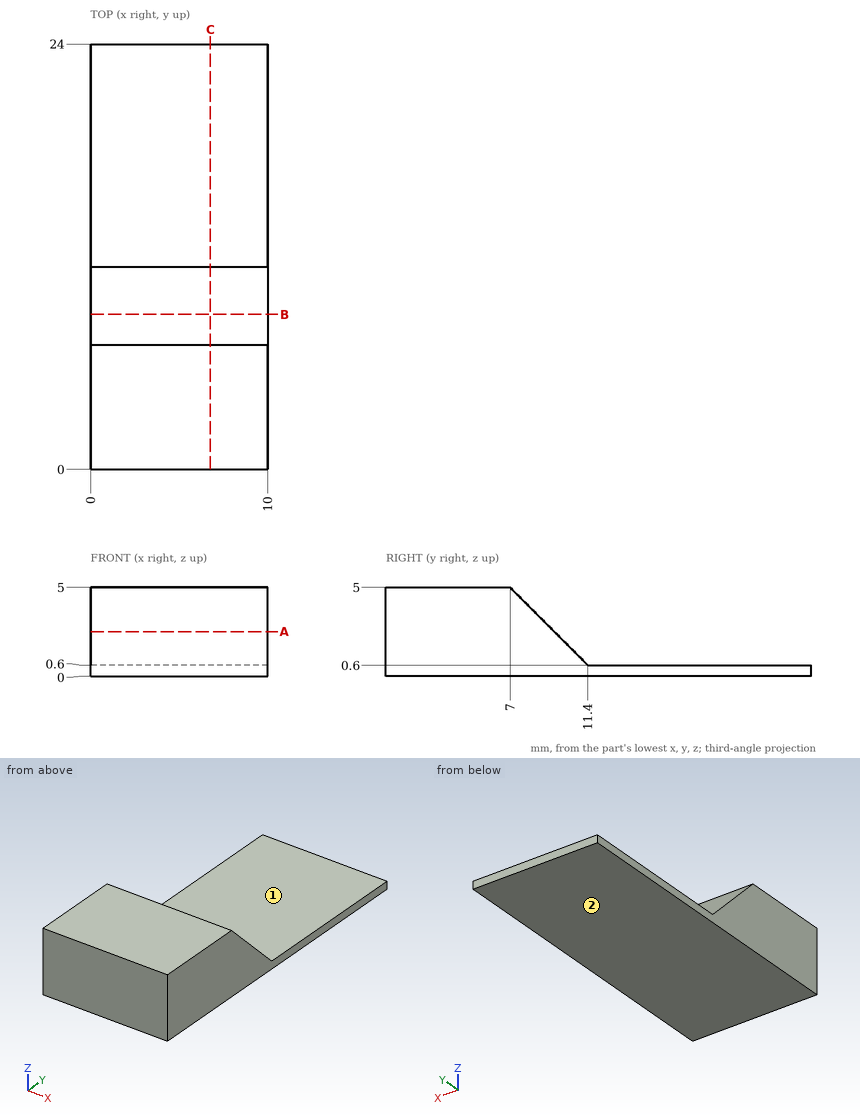
For this review, use the dimensioned drawing (mm, ordinates from the lowest corner) and the shaded views. A direction names the side the tool comes from. Round coordinates to 2 decimals unless told otherwise and drop trailing zeros. Order: outer loops, then holes, each group sorted by start corner. A loop starts at its lowest first (then second) coordinate and runs counter-clockwise, first axis right, second up. Notation, with made-up numbers: M 76,33 L 112,33 A27 cw 112,54 Z; hole C 30,20.25 d10. An arc over 180 degrees is marked long. Use a Markdown table: item, result.
1) Wall thickness on line 1 along Z through (x, y) = (3, 23); line 2 along Y through (x, z) = (7.75, 1.85); line 3 along Y through (x, z) = (1.5, 3.1): over which ranges is each line inside the solid? List them lowest first. Write a range as [from, to].
Report:
| item | result |
|---|---|
| line 1 | [0, 0.6] |
| line 2 | [0, 10.15] |
| line 3 | [0, 8.9] |
2) Consider section A-A (z = 2.5). Write out the cut boundary in (x, y).
Report:
| item | result |
|---|---|
| outline | M 0,0 L 10,0 L 10,9.5 L 0,9.5 Z |
3) Insertion check: pin 1 (5 mm diameter, centred on x = 9, y = 20, fed in from -Z); pin 2 (3 mm diameter, centred on x = 8.5, y = 19, fed in from +Z). Each pin has a flat end and moves straight along its axis. Give the tip position at first contact, or say it passes through.
Report:
| item | result |
|---|---|
| pin 1 | z = 0 |
| pin 2 | z = 0.6 |
4) Consider section B-B (y = 8.75). Write out the cut boundary in (x, z).
Report:
| item | result |
|---|---|
| outline | M 0,0 L 10,0 L 10,3.25 L 0,3.25 Z |
5) Tool access review of the marked faces 1 and 2: name each direction out of +Z, -Z, +X, -X, +Y, -Y from which nothing blocks a thin tool from reaching the whole face with its end or side.
Report:
| item | result |
|---|---|
| face 1 | +Z, +X, -X, +Y |
| face 2 | -Z, +X, -X, +Y, -Y |
6) Consider section C-C (x = 6.75). Write out the cut boundary in (y, z), then the cut area to 3 significant figures.
Report:
| item | result |
|---|---|
| outline | M 0,0 L 24,0 L 24,0.6 L 11.4,0.6 L 7,5 L 0,5 Z |
| area | 54.9 mm^2 |
